```python
from build123d import *

# Parameters (mm, degrees)
SKETCH1_W                 = 44
SKETCH1_H                 = 30
LID_PLATE_DEPTH           = 2
SKETCH2_R                 = 1.45
CLEARANCE_HOLES_DEPTH     = 3
FORWARD_ARROW_X_DEPTH     = 0.6
SKETCH4_W                 = 12
SKETCH4_H                 = 2
BOARD_HOLD_DOWN_RIB_DEPTH = 2.4


with BuildPart() as part:
    # Sketch1 → Lid Plate (new body)
    with BuildSketch(Plane(origin=(0, 0, 0), x_dir=(1, 0, 0), z_dir=(0, 1, 0))):
        Rectangle(SKETCH1_W, SKETCH1_H)
    extrude(amount=LID_PLATE_DEPTH)

    # Sketch2 → Clearance Holes (cut)
    with BuildSketch(Plane(origin=(0, 2, 0), x_dir=(1, 0, 0), z_dir=(0, 1, 0))):
        with Locations(Location((-18, -11, 0), (0, 0, 270))):
            Circle(SKETCH2_R)
        with Locations(Location((-18, 11, 0), (0, 0, 270))):
            Circle(SKETCH2_R)
        with Locations(Location((18, -11, 0), (0, 0, 270))):
            Circle(SKETCH2_R)
        with Locations(Location((18, 11, 0), (0, 0, 270))):
            Circle(SKETCH2_R)
    extrude(amount=-CLEARANCE_HOLES_DEPTH, mode=Mode.SUBTRACT)

    # Sketch3 → Forward Arrow (+X) (cut)
    with BuildSketch(Plane(origin=(0, 2, 0), x_dir=(1, 0, 0), z_dir=(0, 1, 0))):
        Polygon((-9, -1.5), (5, -1.5), (5, -4.5), (11, 0), (5, 4.5), (5, 2.25), (-9, 2.25), align=None)
    extrude(amount=-FORWARD_ARROW_X_DEPTH, mode=Mode.SUBTRACT)

    # Sketch4 → Board Hold-Down Rib (add)
    with BuildSketch(Plane(origin=(0, 0, 0), x_dir=(1, 0, 0), z_dir=(0, 1, 0))):
        with Locations((0, -7)):
            Rectangle(SKETCH4_W, SKETCH4_H)
    extrude(amount=-BOARD_HOLD_DOWN_RIB_DEPTH)


solid = part.part
```
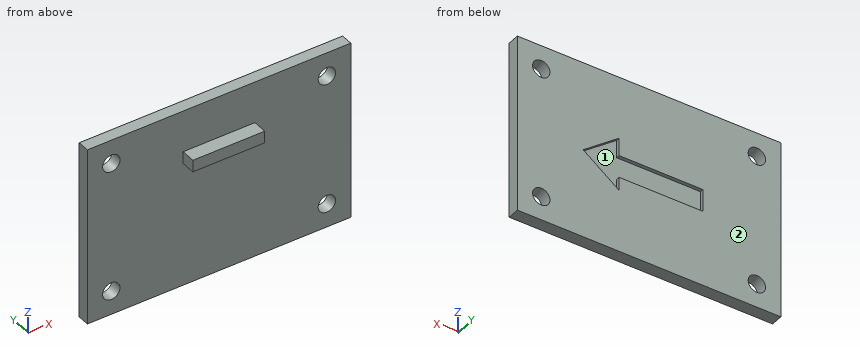
Check sheet for the modelled part. Datum: model origin and axes. Units: mm. Face numbers are marked on the shaded views. Give positions to 0.01 mm unless a question says otherwise; leave off trailing zeros. Order: outer loops, then holes, each group sorted by start corner. A loop starts at its lowest first (then second) coordinate and runs counter-clockwise, first axis right, second up. Notation, with made-up numbers: (-31, 76) -> (1, 76) arc R22 cw to (1, 103) -> close; hole circle Ø5 at (13.5, 25). An arc over 180 degrees is marked (long way). Use CSV: the item, a comma, the result in double quotes. Start each with the question number.
1) Sectioned sample at D-D, the plane z = -6. Record the boundary of the cut face in (x, y), plus the area to 3 significant figures.
2) Sectioned sample at A-A, the plane z = 11. Record the boundary of the cut face in (x, y).
3) Sectioned sample at C-C, the plane x = -8. Record the boundary of the cut face in (y, z).
4) Material ranges on line 1 (X direction, y = 1.2, z = -11); line 2 (X direction, y = 1.8, z = 12.25); line 3 (Y direction, x = -3, z = -12), recorded low to high. Write a range as from..to.
5) Sectioned sample at B-B, the plane x = 18. Record the boundary of the cut face in (y, z).
6) Go/stop test with flat-tipped pins: P1, Ø1, axis at y = -1, z = 7.5, coming from the -X side; P2, Ø1.2, axis at x = 0, y = -1, coming from the -Z side; P3, Ø2.5, axis at x = -18, z = -11, coming from the +Y side; P4, Ø3, axis at x = 9, z = -7, coming from the -Y side. Record where each tip stops, or that it passes through.
7) Mould release check, pull along X, two halves, no side actions. Record for the marked faces 1 and 2: released by +X, released by -X, zero draft, split by the parting line, or undercut.
Recorded:
1,outline,"(-22, 0) -> (22, 0) -> (22, 2) -> (-22, 2) -> close"
1,area,"88.0 mm2"
2,outline,"(-22, 0) -> (-19.45, 0) -> (-19.45, 2) -> (-22, 2) -> close; (-16.55, 0) -> (16.55, 0) -> (16.55, 2) -> (-16.55, 2) -> close; (19.45, 0) -> (22, 0) -> (22, 2) -> (19.45, 2) -> close"
3,outline,"(0, -15) -> (2, -15) -> (2, -2.25) -> (1.4, -2.25) -> (1.4, 1.5) -> (2, 1.5) -> (2, 15) -> (0, 15) -> close"
4,line 1,"-22..-19.45, -16.55..16.55, 19.45..22"
4,line 2,"-22..-18.73, -17.27..17.27, 18.73..22"
4,line 3,"0..2"
5,outline,"(0, -15) -> (2, -15) -> (2, -12.45) -> (0, -12.45) -> close; (0, -9.55) -> (2, -9.55) -> (2, 9.55) -> (0, 9.55) -> close; (0, 12.45) -> (2, 12.45) -> (2, 15) -> (0, 15) -> close"
6,P1,"x = -6"
6,P2,"z = 6"
6,P3,"through"
6,P4,"y = 0"
7,face 1,"undercut"
7,face 2,"zero draft"
